Autodesk Inventor part; units mm, degrees
ref_plane "YZ Plane" through (0, 0, 0) normal (1, 0, 0) x (0, 1, 0)
ref_plane "XZ Plane" through (0, 0, 0) normal (0, 1, 0) x (-1, 0, 0)
ref_plane "XY Plane" through (0, 0, 0) normal (0, 0, 1) x (1, 0, 0)
sketch "Sketch1" plane through (0, 0, 0) normal (0, 0, 1) x (1, 0, 0)
  line L0 (0, 0) -> (43, 0)
  line L1 (43, 0) -> (43, 17.5)
  line L2 (43, 17.5) -> (0, 17.5)
  line L3 (0, 17.5) -> (0, 0)
  dimension "d0" = 43
  dimension "d1" = 17.5
extrude "Extrusion1" add sketch "Sketch1" along normal blind 4
sketch "Sketch2" plane through (0, 0, 4) normal (0, 0, 1) x (1, 0, 0)
  line L0 (0, 0) -> (0, 5)
  line L1 (43, 17.5) -> (0, 17.5)
  line L2 (0, 17.5) -> (0, 12.5)
  line L3 (0, 17.5) -> (0, 0)
  line L4 (0, 12.5) -> (5, 12.5)
  line L5 (5, 12.5) -> (5, 5)
  line L6 (5, 5) -> (0, 5)
  line L7 (0, 12.5) -> (0, 5)
  line L8 (0.0001, 12.5) -> (0.0007, 5)
  dimension "d4" = 5
  dimension "d5" = 5
  dimension "d6" = 5
extrude "Extrusion2" add sketch "Sketch2" along normal blind 8.5
sketch "Sketch3" plane through (0, 0, 4) normal (0, 0, 1) x (1, 0, 0)
  line L0 (43, 0) -> (43, 17.5)
  line L1 (43, 0) -> (43, 5)
  line L2 (43, 5) -> (35.5, 5)
  line L3 (43, 17.5) -> (0, 17.5)
  line L4 (43, 17.5) -> (43, 12.5)
  line L5 (43, 12.5) -> (35.5, 12.5)
  line L6 (35.5, 12.5) -> (35.5, 5)
  point P0 (0, 0)
  dimension "d9" = 5
  dimension "d10" = 7.5
  dimension "d11" = 5
extrude "Extrusion3" add sketch "Sketch3" along normal blind 4
sketch "Sketch4" plane through (43, 0, 0) normal (1, 0, 0) x (0, 0, -1)
  line L0 (-8, 5) -> (-8, 12.5)
  line L1 (-4, 0) -> (-4, 5)
  line L2 (-8, 5) -> (-4, 5)
  line L3 (-4, 5) -> (-4, 12.5)
  line L4 (-4, 12.5) -> (-8, 12.5)
  line L5 (-8, 12.5) -> (-8, 5)
  point P0 (0, 0)
extrude "Extrusion4" add sketch "Sketch4" along normal blind 1.5
properties part number "Arduino Nano"
Verification items for the finished model (mm, model axes). A direction names the side the tool comes from. Coordinates: 2 decimals unless noted, no trailing zeros. Loops run counter-clockwise (first coordinate to the right, second up) from the corner with the lowest first, then second, coordinate; pieces in that order, holes last. Notation, with made-up numbers: (13.25, 28.25) -> (30.25, 28.25) arc R26 ccw to (30.25, 54.25) -> close; hole circle Ø7 at (10, 43.5). An arc over 180 degrees is marked (long way). Put each result on its own line as item: value.
1. Tool access check on faces 5 (the face through (5, 9, 8)), 6 (the face through (2, 12.5, 8)), 7 (the face through (40, 9, 8)), 8 (the face through (3, 5, 8)), 9 (the face through (44, 9, 4)). Record the directions out of +Z, -Z, +X, -X, +Y, -Y that give a thin tool (end or side, any length) a straight path to the whole face; none if there is none.
Result set:
face 5: +Z, +Y, -Y
face 6: +Z, +X, -X, +Y
face 7: +Z, +X, +Y, -Y
face 8: +Z, +X, -X, -Y
face 9: -Z, +X, +Y, -Y
2. Thickness scan on line 1 (X direction, y = 7, z = 7.75); line 2 (X direction, y = 1, z = 0.5); line 3 (Z direction, x = 23.5, y = 10). Record the ranges inside material, lowest first.
Result set:
line 1: x = 0 to 5, 35.5 to 44.5
line 2: x = 0 to 43
line 3: z = 0 to 4
3. Section check C-C, the plane x = 38.5. Record the boundary of the cut face in (y, z), then the cut area to 3 significant figures.
Result set:
outline: (0, 0) -> (17.5, 0) -> (17.5, 4) -> (12.5, 4) -> (12.5, 8) -> (5, 8) -> (5, 4) -> (0, 4) -> close
area: 100 mm^2
4. Section check D-D, the plane z = 1. Record the boundary of the cut face in (x, y), then the cut area to 4 significant figures.
Result set:
outline: (0, 0) -> (43, 0) -> (43, 17.5) -> (0, 17.5) -> close
area: 752.5 mm^2
5. Gauge pin test, flat ends, axial feed: P1, Ø1.2, axis at x = 41.5, z = 6, coming from the -Y side; P2, Ø2, axis at x = 36, y = 15, coming from the +Z side; P3, Ø2.5, axis at x = 2.5, z = 7.5, coming from the +Y side. Record the tip position at first contact, or that the pin passes through.
Result set:
P1: stops at y = 5
P2: stops at z = 4
P3: stops at y = 12.5
6. Mould release check, pull along X, two halves, no side actions. Record for faces 1 (the face through (35.5, 9, 6)), 2 (the face through (21, 9, 4)), 3 (the face through (43, 9, 2)), 4 (the face through (21, 0, 2)): pulls with the +X half, pulls with the -X half, needs draft (parallel to the pull), parting line crosses it, or undercut.
Result set:
face 1: undercut
face 2: undercut
face 3: pulls with the +X half
face 4: needs draft
7. Section check B-B, the plane y = 9.75. Record the boundary of the cut face in (x, z), then the cut area to 4 significant figures.
Result set:
outline: (0, 0) -> (43, 0) -> (43, 4) -> (44.5, 4) -> (44.5, 8) -> (35.5, 8) -> (35.5, 4) -> (5, 4) -> (5, 12.5) -> (0, 12.5) -> close
area: 250.5 mm^2
8. Section check A-A, the plane z = 5.25. Record the boundary of the cut face in (x, y), then the cut area to 3 significant figures.
Result set:
outline: (0, 5) -> (5, 5) -> (5, 12.5) -> (0, 12.5) -> close; (35.5, 5) -> (44.5, 5) -> (44.5, 12.5) -> (35.5, 12.5) -> close
area: 105 mm^2
